Autodesk Inventor part; units mm, degrees
ref_plane "YZ Plane" through (0, 0, 0) normal (1, 0, 0) x (0, 1, 0)
ref_plane "XZ Plane" through (0, 0, 0) normal (0, 1, 0) x (-1, 0, 0)
ref_plane "XY Plane" through (0, 0, 0) normal (0, 0, 1) x (1, 0, 0)
sketch "スケッチ1" plane through (0, 0, 0) normal (0, 0, 1) x (1, 0, 0)
  line L0 (0, 4.5) -> (1.5, 4.5)
  line L1 (1.5, 4.5) -> (1.5, 6)
  line L2 (1.5, 6) -> (3, 6)
  line L3 (3, 6) -> (3, 1.5)
  line L4 (3, 1.5) -> (0, 1.5)
  line L5 (0, -1.2) -> (0, 7.2) construction
  line L6 (0, 4.5) -> (-1.5, 4.5)
  line L7 (-1.5, 4.5) -> (-1.5, 6)
  line L8 (-1.5, 6) -> (-3, 6)
  line L9 (-3, 6) -> (-3, 1.5)
  line L10 (-3, 1.5) -> (0, 1.5)
  line L11 (-4.2, 0) -> (4.2, 0)
  point P0 (0, 0)
  dimension "d0" = 1.5
  dimension "d1" = 4.5
  dimension "d2" = 1.5
  dimension "d3" = 1.5
  dimension "d4" = 1.5
revolve "回転1" add sketch "スケッチ1" angle 360 about axis through (-10, 0, 0) along (1, 0, 0)
properties part number "Pulley_D3_P10"
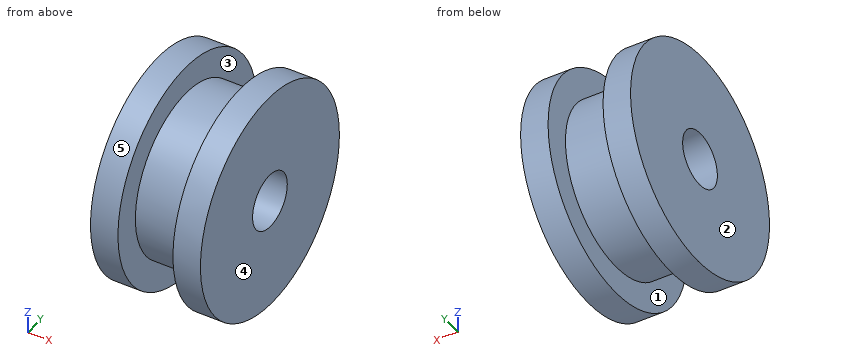
Check sheet for the modelled part. Datum: model origin and axes. Units: mm. Face numbers are marked on the shaded views. A direction names the side the tool comes from. Give positions to 0.01 mm unless a question says otherwise; leave off trailing zeros. Order: outer loops, then holes, each group sorted by start corner. A loop starts at its lowest first (then second) coordinate and runs counter-clockwise, first axis right, second up. Notation, with made-up numbers: (-21.5, -29.5) - (32.5, -29.5) arc R16 cw to (32.5, -10.5) - close; hole circle Ø7 at (51.25, -22). An arc over 180 degrees is marked (long way). Answer as CSV lines item,"result".
1. Scan lines: probe 1 along Z at (x, y) = (1.1, 0); probe 2 along Z at (x, y) = (1.8, 0); probe 3 along X at (y, z) = (3, -4). Record each from-to range of solid material in increasing order. Write a range as from..to.
Result sheet:
probe 1,"-4.5..-1.5, 1.5..4.5"
probe 2,"-6..-1.5, 1.5..6"
probe 3,"-3..-1.5, 1.5..3"
2. Section check A-A (z = 0). Record the boundary of the cut face in (x, y), then the cut area to 3 significant figures.
Result sheet:
outline,"(-3, -6) - (-1.5, -6) - (-1.5, -4.5) - (1.5, -4.5) - (1.5, -6) - (3, -6) - (3, -1.5) - (-3, -1.5) - close; (-3, 1.5) - (3, 1.5) - (3, 6) - (1.5, 6) - (1.5, 4.5) - (-1.5, 4.5) - (-1.5, 6) - (-3, 6) - close"
area,"45.0 mm²"
3. Tool access check on the marked faces 1 and 2. Record the directions out of +Z, -Z, +X, -X, +Y, -Y that give a thin tool (end or side, any length) a straight path to the whole face; none if there is none.
Result sheet:
face 1,"none"
face 2,"+Z, -Z, -X, +Y, -Y"
4. Mould release check, pull along X, two halves, no side actions. Record for the marked faces 3, 4 and 5: released by +X, released by -X, zero draft, split by the parting line, or undercut.
Result sheet:
face 3,"undercut"
face 4,"released by +X"
face 5,"zero draft"
5. Section check C-C (x = 1.8). Record the boundary of the cut face in (y, z), then the cut area to 3 significant figures.
Result sheet:
outline,"circle Ø12 at (0, 0); hole circle Ø3 at (0, 0)"
area,"106 mm²"
6. Section check D-D (y = -3). Record the boundary of the cut face in (x, z).
Result sheet:
outline,"(-3, -5.2) - (-1.5, -5.2) - (-1.5, -3.35) - (1.5, -3.35) - (1.5, -5.2) - (3, -5.2) - (3, 5.2) - (1.5, 5.2) - (1.5, 3.35) - (-1.5, 3.35) - (-1.5, 5.2) - (-3, 5.2) - close"
7. Go/stop test with flat-tipped pins: P1, Ø1, axis at x = -2, y = -4, coming from the +Z side; P2, Ø1.5, axis at x = -0.5, y = -2.5, coming from the -Z side; P3, Ø2, axis at x = 1, z = 4.5, coming from the +Y side. Record where each tip stops, or that it passes through.
Result sheet:
P1,"z = 4.87"
P2,"z = -4.15"
P3,"y = 4.77"
